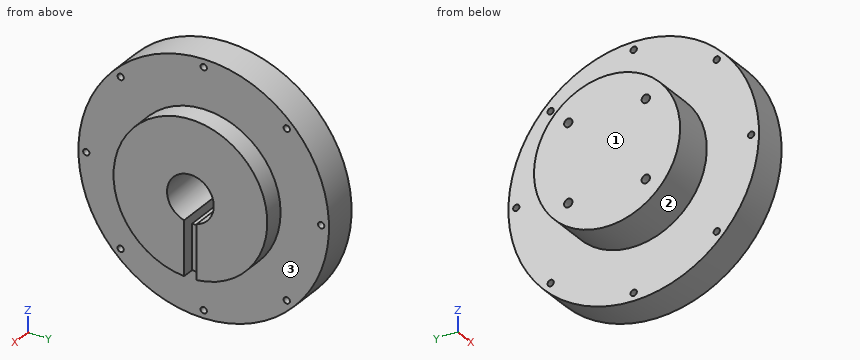
from build123d import *

# Parameters (mm, degrees)
UPPER_CIRLCE_2_R   = 36.83
UPPER_CIRLCE_DEPTH = 10
SKETCH2_R          = 1.5
CUT_EXTRUDE1_DEPTH = 140.185855962
CIRPATTERN1_COUNT  = 8
PIN_SKETCH_R       = 2
CUT_EXTRUDE2_DEPTH = 10
SKETCH3_R          = 11.2
CUT_EXTRUDE3_DEPTH = 29
SKETCH4_W          = 8
SKETCH4_H          = 6
CUT_EXTRUDE4_DEPTH = 70
SKETCH6_W          = 22.346517692
SKETCH6_H          = 6
CUT_EXTRUDE5_DEPTH = 6
SKETCH7_W          = 17.189641189
SKETCH7_H          = 6
CUT_EXTRUDE6_DEPTH = 4


with BuildPart() as part:
    # Sketch1 → Revolve1 (revolve)
    with BuildSketch(Plane.XY, mode=Mode.PRIVATE) as revolve1_sk:
        Polygon((0, 0), (-17, 0), (-17, 25), (-37.05, 25), (-37.05, 60), (0, 60), align=None)
    revolve(revolve1_sk.sketch.rotate(Axis((-37.05, 60, 0), (1, 0, 0)), 270), axis=Axis((-37.05, 60, 0), (1, 0, 0)))

    # upper cirlce 2 → upper cirlce (add)
    with BuildSketch(Plane(origin=(0, 0, 0), x_dir=(0, 0, -1), z_dir=(1, 0, 0))):
        with Locations((0, 60)):
            Circle(UPPER_CIRLCE_2_R)
    extrude(amount=UPPER_CIRLCE_DEPTH)

    # Sketch2 → Cut-Extrude1 (cut, symmetric)
    with BuildSketch(Plane(origin=(0, 0, 0), x_dir=(0, 0, -1), z_dir=(1, 0, 0))):
        with Locations((0, 116.25)):
            Circle(SKETCH2_R)
    cut_extrude1 = extrude(amount=CUT_EXTRUDE1_DEPTH, both=True, mode=Mode.SUBTRACT)

    # CirPattern1: Cut-Extrude1 ×8 about axis
    cirpattern1_axis = Axis((0, 60, 0), (1, 0, 0))
    for i in range(1, CIRPATTERN1_COUNT):
        add(cut_extrude1.rotate(cirpattern1_axis, i * 360 / CIRPATTERN1_COUNT), mode=Mode.SUBTRACT)

    # pin sketch → Cut-Extrude2 (cut)
    with BuildSketch(Plane.ZY.offset(37.05)):
        with Locations((-18.56, 78.56)):
            Circle(PIN_SKETCH_R)
        with Locations((18.56, 78.56)):
            Circle(PIN_SKETCH_R)
        with Locations((18.56, 41.44)):
            Circle(PIN_SKETCH_R)
        with Locations((-18.56, 41.44)):
            Circle(PIN_SKETCH_R)
    extrude(amount=-CUT_EXTRUDE2_DEPTH, mode=Mode.SUBTRACT)

    # Sketch3 → Cut-Extrude3 (cut)
    with BuildSketch(Plane(origin=(10, 0, 0), x_dir=(0, 0, -1), z_dir=(1, 0, 0))):
        with Locations((0, 60)):
            Circle(SKETCH3_R)
    extrude(amount=-CUT_EXTRUDE3_DEPTH, mode=Mode.SUBTRACT)

    # Sketch4 → Cut-Extrude4 (cut)
    with BuildSketch(Plane(origin=(-19, 0, 0), x_dir=(0, 0, -1), z_dir=(1, 0, 0))):
        with Locations((11.2, 60)):
            Rectangle(SKETCH4_W, SKETCH4_H)
    extrude(amount=CUT_EXTRUDE4_DEPTH, mode=Mode.SUBTRACT)

    # Sketch6 → Cut-Extrude5 (cut)
    with BuildSketch(Plane(origin=(10, 0, 0), x_dir=(0, 0, -1), z_dir=(1, 0, 0))):
        with Locations((26.373258846, 60)):
            Rectangle(SKETCH6_W, SKETCH6_H)
    extrude(amount=-CUT_EXTRUDE5_DEPTH, mode=Mode.SUBTRACT)

    # Sketch7 → Cut-Extrude6 (cut)
    with BuildSketch(Plane(origin=(-19, 0, 0), x_dir=(0, 0, -1), z_dir=(1, 0, 0))):
        with Locations((6.605179406, 60)):
            Rectangle(SKETCH7_W, SKETCH7_H)
    extrude(amount=-CUT_EXTRUDE6_DEPTH, mode=Mode.SUBTRACT)


solid = part.part
Verification items for the finished model (mm, model axes). Face numbers are marked on the shaded views. A direction names the side the tool comes from. Give positions to 0.01 mm unless a question says otherwise; leave off trailing zeros. Write each loop counter-clockwise with the first axis right and the second up, starting at its lowest first coordinate (ties: lowest second). Pieces come first, ordered by that corner, then holes. Notation, with made-up numbers: M -17.75,20.25 L -5.75,20.25 A14 ccw -5.75,30.25 Z; hole C 76.25,77 d2. An arc over 180 degrees is marked long. Write item = value, one per line.
(1) Sectioned sample at D-D (z = -56.25). Record the cut outline in (x, y).
Found:
outline = M -17,39.12 L 0,39.12 L 0,58.5 L -17,58.5 Z; M -17,61.5 L 0,61.5 L 0,80.88 L -17,80.88 Z
(2) Material ranges on line 1 (Y direction, x = -10, z = 0); line 2 (Y direction, x = -29, z = -18); line 3 (X direction, y = 98, z = -30), recorded low to high.
Found:
line_1 = 0 to 2.25, 5.25 to 48.8, 71.2 to 114.75, 117.75 to 120
line_2 = 29.98 to 39.52, 43.36 to 76.64, 80.48 to 90.02
line_3 = -17 to 0
(3) Go/stop test with flat-tipped pins: pin 1 Ø2 at (y, z) = (78.5, 19) entering from -X; pin 2 Ø4 at (y, z) = (100, -12) entering from +X; pin 3 Ø1.5 at (y, z) = (83.5, 32) entering from -X. Record where each tip stops, or that it passes through.
Found:
pin_1 = -27.05
pin_2 = 0
pin_3 = -17
(4) Sectioned sample at A-A (z = 0). Record the cut outline in (x, y), then the cut area to 3 significant figures.
Found:
outline = M -37.05,25 L -17,25 L -17,5.25 L 0,5.25 L 0,23.17 L 10,23.17 L 10,48.8 L -19,48.8 L -19,57 L -23,57 L -23,63 L -19,63 L -19,71.2 L 10,71.2 L 10,96.83 L 0,96.83 L 0,114.75 L -17,114.75 L -17,95 L -37.05,95 Z; M -17,0 L 0,0 L 0,2.25 L -17,2.25 Z; M -17,117.75 L 0,117.75 L 0,120 L -17,120 Z
area = 3,400 mm2
(5) Access from +Z, -Z, +X, -X, +Y, -Y to the whole of each face (thin tool, end or side, straight path). Record for the marked faces 1, 2 and 3.
Found:
face_1 = +Z, -Z, -X, +Y, -Y
face_2 = -X
face_3 = +X
(6) Sectioned sample at C-C (y = 3.75). Record the cut outline in (x, z), then the cut area to 3 significant figures.
Found:
outline = M -17,-20.88 L 0,-20.88 L 0,-1.5 L -17,-1.5 Z; M -17,1.5 L 0,1.5 L 0,20.88 L -17,20.88 Z
area = 659 mm2
(7) Sectioned sample at B-B (x = -31). Record the cut outline in (y, z), then the cut area to 3 significant figures.
Found:
outline = C 60,0 d70; hole C 41.44,-18.56 d4; hole C 41.44,18.56 d4; hole C 78.56,-18.56 d4; hole C 78.56,18.56 d4
area = 3,800 mm2
